Model file for the job. Use its own axes, mm. A direction names the side the tool comes from. Coordinates: 2 decimals unless noted, no trailing zeros. Write each loop counter-clockwise with the first axis right and the second up, starting at its lowest first coordinate (ties: lowest second). Pieces come first, ordered by that corner, then holes.
Q1. Pin check, flat tips, straight feed: P1, Ø0.5, axis at x = 0, z = 0, coming from the +Y side; P2, Ø0.7, axis at x = 0, y = 1, coming from the +Z side. Stop position of each tip, or through.
Q2. Which spindle directions (+Z, -Z, +X, -X, +Y, -Y) get a long thin tool onto all of the face, cutting with end or side? Do faces 4 (the flat face through (0, 1, 0.75)), 5 (the cylindrical face through (1, -4, 0)). Say none if no direction does.
Q3. Band-saw the part on A-A, the plane y = -2.75. Write the cut outline in (x, z), plus the area to 3 significant figures.
Q4. Pull direction X, two halves, no side cores. Call faces 1 (the flat face through (0, -7.95, 0)), 2 (the cylindrical face through (1.88, 0.25, -0.42)), 3 (the flat face through (0, 1, -0.75)): released by +X, released by -X, zero draft, split by the parting line, or undercut.
Q5. Drill centre lines: probe 1 along Y at (x, z) = (0.4, -0.2); probe 2 along Z at (x, y) = (-0.35, 1); probe 3 along Y at (x, z) = (-0.3, 1.1). Where is each one in solid material? Low to high.
from build123d import *

# Parameters (mm, degrees)
CUT_EXTRUDE1_DEPTH  = 1.1
BOSS_EXTRUDE1_START = -0.5
SKETCH2_3_R         = 1.309481769
BOSS_EXTRUDE1_DEPTH = 0.267587312


with BuildPart() as part:
    # Sketch1 → Revolve1 (revolve)
    with BuildSketch(Plane(origin=(0, 0, 0), x_dir=(0, 0, -1), z_dir=(1, 0, 0)), mode=Mode.PRIVATE) as revolve1_sk:
        with BuildLine():
            Line((0, -7.95), (0.8, -7.95))
            Line((0.8, -7.95), (1, -7.75))
            Line((1, -7.75), (1, -0.15))
            ThreePointArc((1, -0.15), (1.043933983, -0.043933983), (1.15, 0))
            Line((1.15, 0), (1.925, 0))
            Line((1.925, 0), (1.925, 0.5))
            ThreePointArc((1.925, 0.5), (1.632106781, 1.207106781), (0.925, 1.5))
            Line((0.925, 1.5), (0.8675, 1.5))
            Line((0.8675, 1.5), (0.75, 1.3825))
            Line((0.75, 1.3825), (0.75, 0.5825))
            Line((0.75, 0.5825), (0, 0.381538106))
            Line((0, 0.381538106), (0, -7.95))
        make_face()
    revolve(revolve1_sk.sketch.rotate(Axis((0, 2.837665271, 0), (0, -1, 0)), 180), axis=Axis((0, 2.837665271, 0), (0, -1, 0)))

    # Sketch2 → Cut-Extrude1 (cut)
    with BuildSketch(Plane(origin=(0, 1.5, 0), x_dir=(1, 0, 0), z_dir=(0, 1, 0))):
        Polygon((-0.866025404, 0), (-0.433012702, -0.75), (0.433012702, -0.75), (0.866025404, 0), (0.433012702, 0.75), (-0.433012702, 0.75), align=None)
    extrude(amount=-CUT_EXTRUDE1_DEPTH, mode=Mode.SUBTRACT)

    # Sketch2_3 → Boss-Extrude1 (add)
    with BuildSketch(Plane(origin=(0, 1.5, 0), x_dir=(1, 0, 0), z_dir=(0, 1, 0)).offset(BOSS_EXTRUDE1_START)):
        Circle(SKETCH2_3_R)
        Polygon((0.433012702, -0.75), (0.866025404, 0), (0.433012702, 0.75), (-0.433012702, 0.75), (-0.866025404, 0), (-0.433012702, -0.75), align=None, mode=Mode.SUBTRACT)
    extrude(amount=-BOSS_EXTRUDE1_DEPTH)


solid = part.part
Answer sheet:
1. P1: stops at y = 0.4
1. P2: stops at z = 1.91
2. face 4: +Y
2. face 5: -Y
3. outline: circle Ø2 at (0, 0)
3. area: 3.14 mm2
4. face 1: zero draft
4. face 2: split by the parting line
4. face 3: undercut
5. probe 1: y = -7.95 to 0.4
5. probe 2: z = -1.76 to -0.75, 0.75 to 1.76
5. probe 3: y = 0 to 1.48
